Solid Edge part; units mm, degrees
sketch "Sketch1" plane through (0, 0, 0) normal (0, 0, 1) x (1, 0, 0)
  line L0 (1.5, 0) -> (1.5, 6)
  line L1 (0, 6) -> (1.5, 6)
  line L2 (0, 0) -> (0, 6)
  line L3 (0, 0) -> (0, -1.65)
  line L4 (0, -1.65) -> (2.85, -1.65)
  line L5 (2.85, -1.65) -> (2.85, 0)
  line L6 (2.85, 0) -> (1.5, 0)
revolve "RevolvedProtrusion1" add sketch "Sketch1" angle 360 about axis through (0, 0, 0) along (0, 1, 0)
sketch "Sketch2" plane through (0, 0, 0) normal (1, 0, 0) x (0, 1, 0)
  line L0 (-1.65, 1.6515) -> (-0.61, 1.6515)
  line L1 (0.3435, 0) -> (-0.61, 1.6515)
  line L2 (-1.65, 0) -> (0.3435, 0)
  line L3 (-1.65, 0) -> (-1.65, 1.6515)
revolve "RevolvedCutout1" cut sketch "Sketch2" angle 360 about axis through (0, -4.5, 0) along (0, 1, 0)
sketch "Sketch3" plane through (0, -1.65, 0) normal (0, -1, 0) x (0, 0, 1)
  circle A0 centre (0, 0) radius 1.6515
  line L0 (-1, -0.5774) -> (0, -1.1547)
  line L1 (0, -1.1547) -> (1, -0.5774)
  line L2 (1, -0.5774) -> (1, 0.5774)
  line L3 (1, 0.5774) -> (0, 1.1547)
  line L4 (0, 1.1547) -> (-1, 0.5774)
  line L5 (-1, 0.5774) -> (-1, -0.5774)
extrude "Protrusion1" add sketch "Sketch3" against normal up to next
sketch "Sketch4" plane through (0, 0, 0) normal (0, 0, 1) x (1, 0, 0)
  line L0 (-1.1547, -1.65) -> (0, -1.65)
  line L1 (0, -1.65) -> (0, -1.3406)
  line L2 (0, -1.3406) -> (-1.1547, -1.65)
revolve "RevolvedCutout2" cut sketch "Sketch4" angle 360 about axis through (0, -4.5, 0) along (0, 1, 0)
fillet "Round1" radius 0.1 1 edges at (0, 0, -1.5)
chamfer "倒斜角_2" distance 0.2 angle 45 1 edges at (0, 6, -1.5)
cosmetic_thread "螺纹_3" thread depth 5
sketch "Sketch5" plane through (0, 0, 0) normal (0, 0, 1) x (1, 0, 0)
  arc A0 (-1.5353, -1.65) -> (-2.85, 0) centre (-1.1572, 0) cw
revolve "RevolvedCutout3" cut sketch "Sketch5" angle 360 about axis through (0, 0, 0) along (0, -1, 0) material side at (-2.5202, -1.086, 0)
Could you check a few things on this model? Use its own coordinates, in mm. A direction names the side the tool comes from. Give positions to 0.01 mm unless a question says otherwise; leave off trailing zeros. Order: outer loops, then holes, each group sorted by start corner. A loop starts at its lowest first (then second) coordinate and runs counter-clockwise, first axis right, second up.
1. I need wall thicknesses on L1, parallel to X at y = 5.5, z = 0.75; L2, parallel to Y at x = 2.05, z = 0.35; L3, parallel to Z at x = -0.4, y = 2.5. Which ranges of each line are inside material? Lowest first, please.
Answers below:
L1: x = -1.3 to 1.3
L2: y = -1.42 to 0
L3: z = -1.45 to 1.45
2. Suppose I cut it at A-A (y = 4.5). Write out the boundary of the cut face in (x, z).
Answers below:
outline: circle Ø3 at (0, 0)
3. Thinking about a two-plate mould opening in Z: for faces 3 (the cylindrical face through (-1.5, 2.99, -0.07)), 4 (the flat face through (0, -1, 1)), 5 (the flat face through (0, 0, 2)), which applies, +Z half, -Z half, draft (parallel to the pull), parting line (faces both ways), or undercut?
Answers below:
face 3: parting line
face 4: undercut
face 5: draft
4. Which directions (+Z, -Z, +X, -X, +Y, -Y) give clear straight access to the entire face, cutting with the end or side of a thin tool? Please do faces 1 (the flat face through (0, -1, -1)), 2 (the flat face through (0, 6, 0)).
Answers below:
face 1: -Y
face 2: +Z, -Z, +X, -X, +Y
5. For pin 1 (2 mm diameter, centred on x = 1, z = -1, fed in from +Y); pin 2 (1 mm diameter, centred on y = 2, z = 0, fed in from -X); pin 3 (1.5 mm diameter, centred on y = 4, z = 1.5, fed in from +X); pin 4 (0.6 mm diameter, centred on x = 0, y = -1, fed in from +Z), each with a flat end and sliding along its axis, tell me the tip position at first contact or that it passes through.
Answers below:
pin 1: stops at y = 6
pin 2: stops at x = -1.5
pin 3: stops at x = 1.3
pin 4: stops at z = 2.7
